The model under review builds one solid part; all positions refer to its coordinate system, in mm. Coordinates: 2 decimals unless noted, no trailing zeros. Order: outer loops, then holes, each group sorted by start corner. A loop starts at its lowest first (then second) coordinate and runs counter-clockwise, first axis right, second up. Notation, with made-up numbers: (85.25, 60.5) - (107.25, 60.5) arc R37 ccw to (107.25, 96.5) - close; hole circle Ø9 at (13, -31.75). An arc over 180 degrees is marked (long way). Answer in a Markdown table with one row per item.
```python
from build123d import *

# Parameters (mm, degrees)
BOSS_EXTRUDE2_DEPTH = 6
FILLET1_R           = 3


with BuildPart() as part:
    # Sketch1 → Boss-Extrude2 (new body)
    with BuildSketch(Plane.XY):
        with BuildLine():
            Line((-75, 0), (-69, 0))
            ThreePointArc((-69, 0), (0, -69), (69, 0))
            Line((69, 0), (75, 0))
            ThreePointArc((75, 0), (0, -75), (-75, 0))
        make_face()
    extrude(amount=-BOSS_EXTRUDE2_DEPTH)

    # Fillet1
    fillet1_edges = [part.edges().sort_by_distance(p)[0] for p in [
        (0, -69, -6),
        (0, -69, 0),
        (0, -75, -6),
        (0, -75, 0),
    ]]
    fillet(fillet1_edges, radius=FILLET1_R - 0.0001)  # a hair under: the kernel refuses the full size


solid = part.part
```
Item 1: Clearance check with flat-ended pins moving along their axes: pin 1 Ø3 at (x, z) = (-17.5, -1) entering from -Y; pin 2 Ø1.5 at (x, y) = (39, -63.5) entering from +Z. State where each tip first meets the part, or that it passes through.
Check values:
| item | result |
|---|---|
| pin 1 | y = -73.03 |
| pin 2 | z = -0.58 |
Item 2: To check wall thickness, follow line 1 (X direction, y = -44, z = -1.5); line 2 (X direction, y = -50, z = -2.25); line 3 (Y direction, x = -7, z = -4.25). State the ranges of each line that lie inside material, in increasing order. Write a range as from..to.
Check values:
| item | result |
|---|---|
| line 1 | -60.24..-53.67, 53.67..60.24 |
| line 2 | -55.77..-47.69, 47.69..55.77 |
| line 3 | -74.4..-68.92 |
Item 3: We need section A-A, the plane z = -2. Write out the cut boundary in (x, y).
Check values:
| item | result |
|---|---|
| outline | (-74.83, 0) arc R74.83 ccw to (74.83, 0) - (69.17, 0) arc R69.17 cw to (-69.17, 0) - close |
